Verification items for the finished model (mm, model axes). Face numbers are marked on the shaded views. A direction names the side the tool comes from. Coordinates: 2 decimals unless noted, no trailing zeros. Write each loop counter-clockwise with the first axis right and the second up, starting at its lowest first coordinate (ties: lowest second). Pieces come first, ordered by that corner, then holes. Notation, with made-up numbers: (77, 41.5) -> (120, 41.5) arc R11 ccw to (120, 47.5) -> close; hole circle Ø11 at (-10.5, 77). An arc over 180 degrees is marked (long way). Answer in a Markdown table with one row per item.
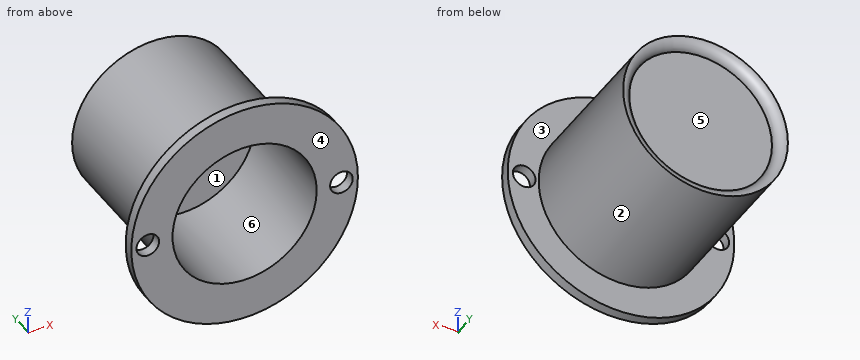
```python
from build123d import *

# Parameters (mm, degrees)
SKETCH_2_R          = 7
CUT_EXTRUDE_1_DEPTH = 10
SKETCH_3_R          = 11
SKETCH_3_R_2        = 7
EXTRUDE_1_DEPTH     = 1
SKETCH_4_R          = 1.1
CUT_EXTRUDE_2_DEPTH = 1


with BuildPart() as part:
    # 草图1 → 旋转1 (revolve)
    with BuildSketch(Plane.XY):
        with BuildLine():
            Line((0, 14), (-7, 14))
            ThreePointArc((-7, 14), (-7.292893219, 14.707106781), (-8, 15))
            Line((-8, 15), (-8, 0))
            Line((-8, 0), (0, 0))
            Line((0, 0), (0, 14))
        make_face()
    revolve(axis=Axis((0, 0, 0), (0, 1, 0)))

    # 草图2 → 切除-拉伸1 (cut)
    with BuildSketch(Plane.XZ):
        Circle(SKETCH_2_R)
    extrude(amount=-CUT_EXTRUDE_1_DEPTH, mode=Mode.SUBTRACT)

    # 草图3 → 凸台-拉伸1 (add)
    with BuildSketch(Plane.XZ):
        Circle(SKETCH_3_R)
        Circle(SKETCH_3_R_2, mode=Mode.SUBTRACT)
    extrude(amount=EXTRUDE_1_DEPTH)

    # 草图4 → 切除-拉伸2 (cut)
    with BuildSketch(Plane.XZ.offset(1)):
        with Locations((9.4, 0)):
            Circle(SKETCH_4_R)
        with Locations((-9.4, 0)):
            Circle(SKETCH_4_R)
    extrude(amount=-CUT_EXTRUDE_2_DEPTH, mode=Mode.SUBTRACT)


solid = part.part
```
1. Sectioned sample at A-A, the plane z = 0. Record the cut outline in (x, y).
Findings below:
| item | result |
|---|---|
| outline | (-11, -1) -> (-10.5, -1) -> (-10.5, 0) -> (-11, 0) -> close; (-8.3, -1) -> (-7, -1) -> (-7, 10) -> (7, 10) -> (7, -1) -> (8.3, -1) -> (8.3, 0) -> (8, 0) -> (8, 15) arc R1 ccw to (7, 14) -> (-7, 14) arc R1 ccw to (-8, 15) -> (-8, 0) -> (-8.3, 0) -> close; (10.5, -1) -> (11, -1) -> (11, 0) -> (10.5, 0) -> close |
2. Sectioned sample at D-D, the plane y = 4.5. Record the cut outline in (x, z).
Findings below:
| item | result |
|---|---|
| outline | circle Ø16 at (0, 0); hole circle Ø14 at (0, 0) |
3. Sectioned sample at C-C, the plane x = 9.4. Record the cut outline in (y, z).
Findings below:
| item | result |
|---|---|
| outline | (-1, -5.71) -> (0, -5.71) -> (0, -1.1) -> (-1, -1.1) -> close; (-1, 1.1) -> (0, 1.1) -> (0, 5.71) -> (-1, 5.71) -> close |
4. Go/stop test with flat-tipped pins: pin 1 (1 mm diameter, centred on x = -2, y = 1.5, fed in from -Z); pin 2 (3 mm diameter, centred on x = -5.5, y = 2.5, fed in from +Z); pin 3 (4 mm diameter, centred on x = 2, z = 0.5, fed in from -Y). Record where each tip stops, or that it passes through.
Findings below:
| item | result |
|---|---|
| pin 1 | stops at z = -7.86 |
| pin 2 | stops at z = 6.93 |
| pin 3 | stops at y = 10 |
5. Release check for a two-part mould opening along X. For the marked faces 1, 2 and 3 record: released by +X, released by -X, zero draft, split by the parting line, or undercut.
Findings below:
| item | result |
|---|---|
| face 1 | undercut |
| face 2 | split by the parting line |
| face 3 | zero draft |
6. Access from +Z, -Z, +X, -X, +Y, -Y to the whole of each face (thin tool, end or side, straight path). Record for the marked faces 4, 5 and 6.
Findings below:
| item | result |
|---|---|
| face 4 | +Z, -Z, +X, -X, -Y |
| face 5 | +Y |
| face 6 | -Y |
7. Material ranges on probe 1 along Z at (x, y) = (0.25, 8.5); probe 2 along X at (y, z) = (13.5, -0.25); probe 3 along Y at (x, z) = (-1, -6.25), recorded low to high. Write a range as from..to.
Findings below:
| item | result |
|---|---|
| probe 1 | z = -8..-7, 7..8 |
| probe 2 | x = -8..8 |
| probe 3 | y = 10..14 |
8. Sectioned sample at B-B, the plane x = 0. Record the cut outline in (y, z).
Findings below:
| item | result |
|---|---|
| outline | (-1, -11) -> (0, -11) -> (0, -8) -> (15, -8) arc R1 ccw to (14, -7) -> (14, 7) arc R1 ccw to (15, 8) -> (0, 8) -> (0, 11) -> (-1, 11) -> (-1, 7) -> (10, 7) -> (10, -7) -> (-1, -7) -> close |
